The listing builds one solid part. Answer for the finished solid, in the listing's coordinates (mm). A direction names the side the tool comes from. Coordinates: 2 decimals unless noted, no trailing zeros.
```python
from build123d import *

# Parameters (mm, degrees)
F0_R      = 2.25
F1_DEPTH  = 5
F3_DEPTH  = 34
F3_TAPER  = 1
F4_R      = 27
F5_DEPTH  = 2.2
F6_R      = 22.5
F7_DEPTH  = 1.2
F7_TAPER  = 60
F8_R      = 4.65
F9_DEPTH  = 5
F10_R     = 3.375
F11_DEPTH = 20


with BuildPart() as f1:
    # F0 (on Front) → F1 (new body)
    with BuildSketch(Plane.XZ):
        with BuildLine():
            ThreePointArc((30, 25), (28.5355339059, 28.5355339059), (25, 30))
            Line((25, 30), (-25, 30))
            ThreePointArc((-25, 30), (-28.5355339059, 28.5355339059), (-30, 25))
            Line((-30, 25), (-30, -25))
            ThreePointArc((-30, -25), (-28.5355339059, -28.5355339059), (-25, -30))
            Line((-25, -30), (25, -30))
            ThreePointArc((25, -30), (28.5355339059, -28.5355339059), (30, -25))
            Line((30, -25), (30, 25))
        make_face()
        with Locations((-24.75, -24.75)):
            Circle(F0_R, mode=Mode.SUBTRACT)
        with Locations((24.75, -24.75)):
            Circle(F0_R, mode=Mode.SUBTRACT)
        with Locations((-24.75, 24.75)):
            Circle(F0_R, mode=Mode.SUBTRACT)
        with Locations((24.75, 24.75)):
            Circle(F0_R, mode=Mode.SUBTRACT)
    extrude(amount=-F1_DEPTH)

    # F2 (on face) → F3 (join)
    with BuildSketch(Plane(origin=(0, 5, 0), x_dir=(-1, 0, 0), z_dir=(0, 1, 0))):
        with BuildLine():
            Line((-16.1994765079, -28.5), (16.1994765079, -28.5))
            ThreePointArc((16.1994765079, -28.5), (17.5376209063, -27.9863948227), (18.1884874138, -26.709369569))
            Line((18.1884874138, -26.709369569), (18.6610206978, -22.2203033714))
            ThreePointArc((18.6610206978, -22.2203033714), (19.8106153847, -19.8106153847), (22.2203033714, -18.6610206978))
            Line((22.2203033714, -18.6610206978), (26.709369569, -18.1884874138))
            ThreePointArc((26.709369569, -18.1884874138), (27.9863948227, -17.5376209063), (28.5, -16.1994765079))
            Line((28.5, -16.1994765079), (28.5, 16.1994765079))
            ThreePointArc((28.5, 16.1994765079), (27.9863948227, 17.5376209063), (26.709369569, 18.1884874138))
            Line((26.709369569, 18.1884874138), (22.2203033714, 18.6610206978))
            ThreePointArc((22.2203033714, 18.6610206978), (19.8106153847, 19.8106153847), (18.6610206978, 22.2203033714))
            Line((18.6610206978, 22.2203033714), (18.1884874138, 26.709369569))
            ThreePointArc((18.1884874138, 26.709369569), (17.5376209063, 27.9863948227), (16.1994765079, 28.5))
            Line((16.1994765079, 28.5), (-16.1994765079, 28.5))
            ThreePointArc((-16.1994765079, 28.5), (-17.5376209063, 27.9863948227), (-18.1884874138, 26.709369569))
            Line((-18.1884874138, 26.709369569), (-18.6610206978, 22.2203033714))
            ThreePointArc((-18.6610206978, 22.2203033714), (-19.8106153847, 19.8106153847), (-22.2203033714, 18.6610206978))
            Line((-22.2203033714, 18.6610206978), (-26.709369569, 18.1884874138))
            ThreePointArc((-26.709369569, 18.1884874138), (-27.9863948227, 17.5376209063), (-28.5, 16.1994765079))
            Line((-28.5, 16.1994765079), (-28.5, -16.1994765079))
            ThreePointArc((-28.5, -16.1994765079), (-27.9863948227, -17.5376209063), (-26.709369569, -18.1884874138))
            Line((-26.709369569, -18.1884874138), (-22.2203033714, -18.6610206978))
            ThreePointArc((-22.2203033714, -18.6610206978), (-19.8106153847, -19.8106153847), (-18.6610206978, -22.2203033714))
            Line((-18.6610206978, -22.2203033714), (-18.1884874138, -26.709369569))
            ThreePointArc((-18.1884874138, -26.709369569), (-17.5376209063, -27.9863948227), (-16.1994765079, -28.5))
        make_face()
    extrude(amount=F3_DEPTH, taper=F3_TAPER)

    # F4 (on face) → F5 (join)
    with BuildSketch(Plane.XZ):
        Circle(F4_R)
    extrude(amount=F5_DEPTH)

    # F6 (on face) → F7 (cut)
    with BuildSketch(Plane.XZ.offset(2.2)):
        Circle(F6_R)
    extrude(amount=-F7_DEPTH, taper=F7_TAPER, mode=Mode.SUBTRACT)

    # F8 (on face) → F9 (cut)
    with BuildSketch(Plane.XZ.offset(1)):
        Circle(F8_R)
    extrude(amount=-F9_DEPTH, mode=Mode.SUBTRACT)

    # F10 (on face) → F11 (join)
    with BuildSketch(Plane.XZ.offset(-4)):
        Circle(F10_R)
    extrude(amount=F11_DEPTH)


solid = f1.part
```
(1) Consider line 1 (Z direction, x = 24.75, y = 3.3); line 2 (Y direction, x = -27, z = -12.5); line 3 (Y direction, x = 24.5, z = 7.5). Determine where each line is inside the solid, lowest interval first.
(2) The mould has two halves that part along X. Classify faces 5 (the face through (-0.7, -5.9, -3.3)), 6 (the face through (-28, 2, 29)), 7 (the face through (17.323, 22.238, 27.774)): released by +X, released by -X, zero draft, split by the parting line, or undercut.
(3) For faces 1 (the face through (-5, 5, -29)), 2 (the face through (2, 4, 3)), 3 (the face through (-19.569, 22.238, -19.627)), 4 (the face through (-17.35, 22.24, 27.75)), determine the directions among +Z, -Z, +X, -X, +Y, -Y from which every point of the face is accessible in a straight line to the end or side of a thin tool.
(4) Each of these flat-tipped pins is pushed along its axis until it touches: pin 1 Ø12 at (y, z) = (30, 8) entering from +X; pin 2 Ø3.5 at (x, z) = (24.75, -24.75) entering from +Y; pin 3 Ø8 at (x, z) = (-15, -11) entering from -Y; pin 4 Ø12 at (x, y) = (3.5, 8) entering from +Z. Where does it stop, or does it pass through?
Findings below:
1. line 1: z = -30 to -27, -22.5 to 22.5, 27 to 30
1. line 2: y = 0 to 39
1. line 3: y = -2.2 to 39
2. face 5: undercut
2. face 6: released by -X
2. face 7: released by +X
3. face 1: +Y
3. face 2: -Y
3. face 3: -Z, -X, +Y
3. face 4: +Z, -X, +Y
4. pin 1: stops at x = 28.17
4. pin 2: passes through
4. pin 3: stops at y = -2.2
4. pin 4: stops at z = 30
